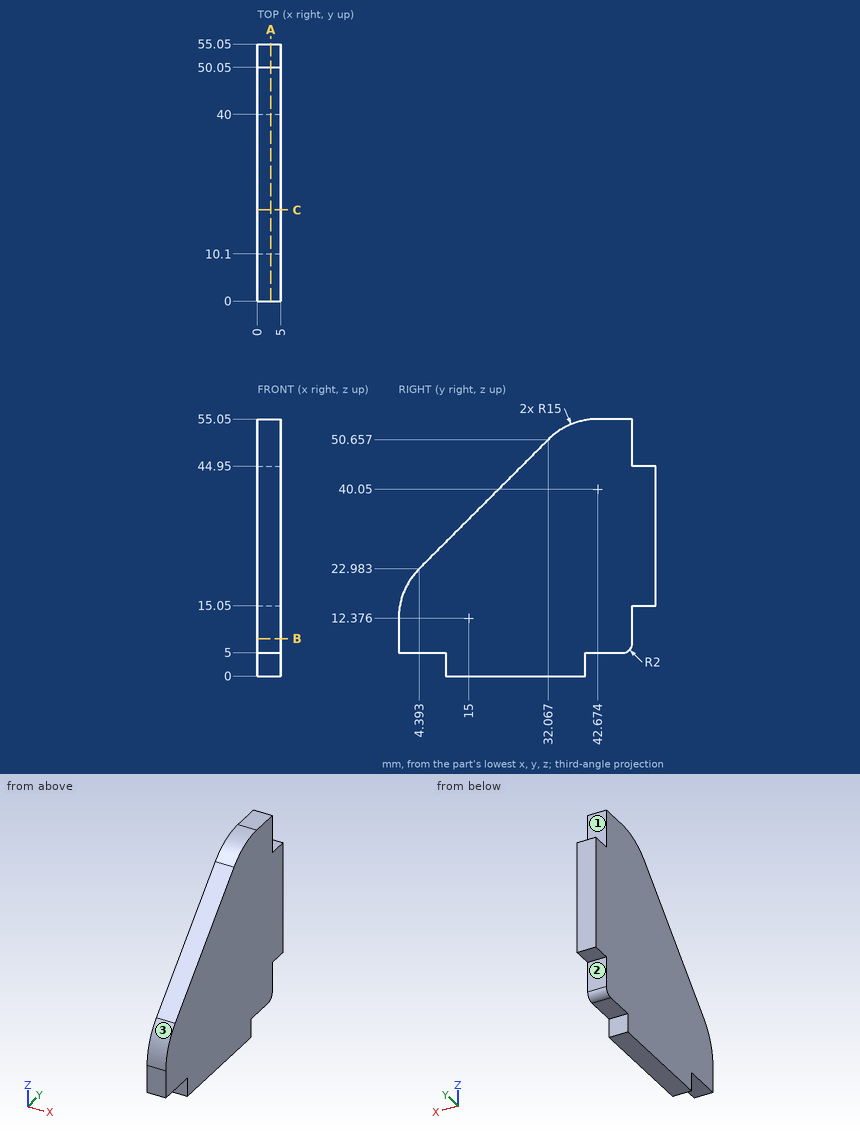
Geometry check sheet. Reference: drawing and pictorial views, mm from the part's lowest x, y, z. A direction names the side the tool comes from. Coordinates: 2 decimals unless noted, no trailing zeros. Order: outer loops, then holes, each group sorted by start corner. A loop starts at its lowest first (then second) coordinate and runs counter-clockwise, first axis right, second up.
Item 1: Section check A-A (x = 2.9). Enter the section's corners in (y, z).
Item 2: Section check B-B (z = 8). Enter the section's corners in (x, y).
Item 3: Section check C-C (y = 19.5). Enter the section's corners in (x, z).
Item 4: Depth check by flat-ended pin: pin 1 (3 mm diameter, centred on y = 13, z = 35, fed in from -X); pin 2 (2.5 mm diameter, centred on x = 3.5, z = 1.5, fed in from +Y); pin 3 (2.5 mm diameter, centred on x = 1.5, y = 53, fed in from +Z); pin 4 (1.5 mm diameter, centred on x = 3.5, z = 3.5, fed in from -Y). Enter the tip coordinate at first touch or a pass-through.
Item 5: Scan lines: line 1 along Y through (x, z) = (1.1, 4); line 2 along Y through (x, z) = (3.65, 12.5); line 3 along Z through (x, y) = (2.8, 33.5). Record each from-to range of solid material in increasing order.
Item 6: Tool access check on the marked faces 1, 2 and 3. Record the directions out of +Z, -Z, +X, -X, +Y, -Y that give a thin tool (end or side, any length) a straight path to the whole face; none if there is none.
Check sheet entries:
1. outline: (0, 5) - (10.1, 5) - (10.1, 0) - (40, 0) - (40, 5) - (48.05, 5) arc R2 ccw to (50.05, 7) - (50.05, 15.05) - (55.05, 15.05) - (55.05, 44.95) - (50.05, 44.95) - (50.05, 55.05) - (42.67, 55.05) arc R15 ccw to (32.07, 50.66) - (4.39, 22.98) arc R15 ccw to (0, 12.38) - close
2. outline: (0, 0) - (5, 0) - (5, 50.05) - (0, 50.05) - close
3. outline: (0, 0) - (5, 0) - (5, 38.09) - (0, 38.09) - close
4. pin 1: passes through
4. pin 2: stops at y = 40
4. pin 3: stops at z = 44.95
4. pin 4: stops at y = 10.1
5. line 1: y = 10.1 to 40
5. line 2: y = 0 to 50.05
5. line 3: z = 0 to 51.92
6. face 1: +Z, +X, -X, +Y
6. face 2: -Z, +X, -X, +Y
6. face 3: +Z, +X, -X, -Y
